Autodesk Inventor part; units mm, degrees
ref_plane "YZ Plane" through (0, 0, 0) normal (1, 0, 0) x (0, 1, 0)
ref_plane "XZ Plane" through (0, 0, 0) normal (0, 1, 0) x (-1, 0, 0)
ref_plane "XY Plane" through (0, 0, 0) normal (0, 0, 1) x (1, 0, 0)
sketch "Sketch1" plane through (0, 0, 0) normal (0, 1, 0) x (-1, 0, 0)
  circle A0 centre (0, 0) radius 12.5
  line L0 (11.7462, -4.2753) -> (40, -14.5588)
  line L1 (0, 0) -> (41.7481, 0) construction
  line L2 (0, 0) -> (11.7462, -4.2753) construction
  line L3 (0, 0) -> (0, -75)
  line L4 (0, -75) -> (27.0598, -66.8927) construction
  line L5 (27.0598, -66.8927) -> (47.507, -49.1207) construction
  line L6 (47.507, -49.1207) -> (40, -14.5588) construction
  spline S0 degree 3 poles (0, -75) (27.0598, -66.8927) (47.507, -49.1207) (40, -14.5588) knots 1 1 1 1 2 2 2 2
  point P0 (0, -12.5)
  dimension "d0" = 25
  dimension "d1" = 40
  dimension "d3" = 20
  dimension "d4" = 75
extrude "Extrusion1" add sketch "Sketch1" along normal blind 2
sketch "Sketch2" plane through (0, 0, 0) normal (0, -1, 0) x (1, 0, 0)
  circle A0 centre (0, 0) radius 2.5
  dimension "d7" = 5
extrude "Extrusion2" add sketch "Sketch2" along normal blind 10
sketch "Sketch4" plane through (0, 0, 0) normal (0, -1, 0) x (1, 0, 0)
  circle A0 centre (-33.6672, -19.171) radius 1.25
  circle A1 centre (-5, -65) radius 1.25
  point P0 (0, 0)
extrude "Extrusion4" cut sketch "Sketch4" against normal up to surface (2 mm away)
properties part number "clamshell half" material "ABS Plastic"
Model file for the job. Use its own axes, mm. A direction names the side the tool comes from. Round coordinates to 2 decimals unless told otherwise and drop trailing zeros. Loops run counter-clockwise (first coordinate to the right, second up) from the corner with the lowest first, then second, coordinate; pieces in that order, holes last.
1. Tool access for faces 4 (the flat face through (0, 1, -43)), 5 (the cylindrical face through (-33.9, 1, -20.4)): list every direction of +Z, -Z, +X, -X, +Y, -Y with a clear straight run to the whole face (end or side of a thin tool).
Check values:
face 4: -Z, +X, +Y, -Y
face 5: +Y, -Y
2. Mould opens along Z. For faces 1 (the cylindrical face through (-5.16, 0.99, -63.76)), 2 (the flat face through (-17, 0, -31)), 3 (the cylindrical face through (-0.54, -4.93, 2.44)) say: +Z half, -Z half, draft (parallel to the pull), parting line (faces both ways), or undercut.
Check values:
face 1: undercut
face 2: draft
face 3: parting line
3. Band-saw the part on B-B, the plane y = -7.25. List the corners of the cut face in (x, z), and give its area (3 significant figures).
Check values:
outline: circle Ø5 at (0, 0)
area: 19.6 mm2
4. Band-saw the part on A-A, the plane z = 0. List the corners of the cut face in (x, y).
Check values:
outline: (-12.5, 0) - (-2.5, 0) - (-2.5, -10) - (2.5, -10) - (2.5, 0) - (12.5, 0) - (12.5, 2) - (-12.5, 2) - close
5. Band-saw the part on C-C, the plane x = 6. List the corners of the cut face in (y, z), and give its area (3 significant figures).
Check values:
outline: (0, -10.97) - (2, -10.97) - (2, 10.97) - (0, 10.97) - close
area: 43.9 mm2
6. Wall check: probe 1 along Y at (x, z) = (-32, -42); probe 2 along Z at (x, y) = (0, -3.75); probe 3 along Z at (x, y) = (-5, 0.55). Give the ranges that are in metal, low to high.
Check values:
probe 1: y = 0 to 2
probe 2: z = -2.5 to 2.5
probe 3: z = -73.36 to -66.25, -63.75 to 11.46
7. Drop flat-ended pins along their axis: P1, Ø6, axis at x = -6, z = -23.5, coming from the -Y side; P2, Ø6, axis at y = 0, z = 1.5, coming from the -X side; P3, Ø1.6, axis at y = 1, z = -42, coming from the +X side. Give the stop position or say it passes through.
Check values:
P1: stops at y = 0
P2: stops at x = -12.5
P3: stops at x = 0
